The listing builds one solid part. Answer for the finished solid, in the listing's coordinates (mm). A direction names the side the tool comes from. Give positions to 0.01 mm unless a question says otherwise; leave off trailing zeros. Write each loop counter-clockwise with the first axis right and the second up, starting at its lowest first coordinate (ties: lowest second). Pieces come first, ordered by that corner, then holes. Notation, with made-up numbers: (71, -37.5) -> (96, -37.5) arc R12 ccw to (96, -30.5) -> close; hole circle Ø11 at (24.5, 50). An arc over 180 degrees is marked (long way). One line per question, with ' | ' between items.
from build123d import *

# Parameters (mm, degrees)
SKETCH1_W           = 43
SKETCH1_H           = 21
BOSS_EXTRUDE1_DEPTH = 1.2
SKETCH2_R           = 0.5
CUT_EXTRUDE1_DEPTH  = 48.868987873
SKETCH3_R           = 1.5
CUT_EXTRUDE2_DEPTH  = 48.868987873
SKETCH4_W           = 9.5
SKETCH4_H           = 4.82
BOSS_EXTRUDE2_DEPTH = 11.88
SKETCH5_R           = 1.12
BOSS_EXTRUDE3_DEPTH = 1.6
SKETCH6_W           = 7.46
SKETCH6_H           = 2.45
BOSS_EXTRUDE4_DEPTH = 0.6
SKETCH7_W           = 12.24
SKETCH7_H           = 12.24
BOSS_EXTRUDE5_DEPTH = 7.61
SKETCH8_W           = 10.2
SKETCH8_H           = 12.8
BOSS_EXTRUDE6_DEPTH = 5.8
SKETCH9_W           = 5.4
SKETCH9_H           = 2.7
BOSS_EXTRUDE7_DEPTH = 2.05
SKETCH10_R          = 4.12
BOSS_EXTRUDE8_DEPTH = 10.3
SKETCH11_R          = 4
BOSS_EXTRUDE9_DEPTH = 10.5


with BuildPart() as part:
    # Sketch1 → Boss-Extrude1 (new body)
    with BuildSketch(Plane(origin=(0, 0, 0), x_dir=(1, 0, 0), z_dir=(0, 1, 0))):
        with Locations((21.5, 10.5)):
            Rectangle(SKETCH1_W, SKETCH1_H)
    extrude(amount=BOSS_EXTRUDE1_DEPTH)

    # Sketch2 → Cut-Extrude1 (cut, through all)
    with BuildSketch(Plane(origin=(0, 1.2, 0), x_dir=(1, 0, 0), z_dir=(0, 1, 0))):
        with Locations(Location((1.4, 19.3, 0), (0, 0, 270))):
            Circle(SKETCH2_R)
        with Locations(Location((1.4, 1.5, 0), (0, 0, 270))):
            Circle(SKETCH2_R)
        with Locations(Location((41.6, 19.3, 0), (0, 0, 270))):
            Circle(SKETCH2_R)
        with Locations(Location((41.6, 1.5, 0), (0, 0, 270))):
            Circle(SKETCH2_R)
    extrude(amount=-CUT_EXTRUDE1_DEPTH, mode=Mode.SUBTRACT)

    # Sketch3 → Cut-Extrude2 (cut, through all)
    with BuildSketch(Plane(origin=(0, 1.2, 0), x_dir=(1, 0, 0), z_dir=(0, 1, 0))):
        with Locations(Location((5.9, 18.94, 0), (0, 0, 270))):
            Circle(SKETCH3_R)
        with Locations(Location((37.05, 2.23, 0), (0, 0, 270))):
            Circle(SKETCH3_R)
    extrude(amount=-CUT_EXTRUDE2_DEPTH, mode=Mode.SUBTRACT)

    # Sketch4 → Boss-Extrude2 (add)
    with BuildSketch(Plane(origin=(0, 1.2, 0), x_dir=(1, 0, 0), z_dir=(0, 1, 0))):
        with Locations((28.93, 18.49)):
            Rectangle(SKETCH4_W, SKETCH4_H)
    extrude(amount=BOSS_EXTRUDE2_DEPTH)

    # Sketch5 → Boss-Extrude3 (add)
    with BuildSketch(Plane(origin=(0, 13.08, 0), x_dir=(1, 0, 0), z_dir=(0, 1, 0))):
        with Locations(Location((25.3, 19.78, 0), (0, 0, 90))):
            Circle(SKETCH5_R)
    extrude(amount=BOSS_EXTRUDE3_DEPTH)

    # Sketch6 → Boss-Extrude4 (add)
    with BuildSketch(Plane.XZ):
        with Locations((29.47, -18.275)):
            Rectangle(SKETCH6_W, SKETCH6_H)
    extrude(amount=BOSS_EXTRUDE4_DEPTH)

    # Sketch7 → Boss-Extrude5 (add)
    with BuildSketch(Plane(origin=(0, 1.2, 0), x_dir=(1, 0, 0), z_dir=(0, 1, 0))):
        with Locations((27.32, 6.87)):
            Rectangle(SKETCH7_W, SKETCH7_H)
    extrude(amount=BOSS_EXTRUDE5_DEPTH)

    # Sketch8 → Boss-Extrude6 (add)
    with BuildSketch(Plane(origin=(0, 1.2, 0), x_dir=(1, 0, 0), z_dir=(0, 1, 0))):
        with Locations((15.3, 13.5)):
            Rectangle(SKETCH8_W, SKETCH8_H)
    extrude(amount=BOSS_EXTRUDE6_DEPTH)

    # Sketch9 → Boss-Extrude7 (add)
    with BuildSketch(Plane(origin=(0, 1.2, 0), x_dir=(1, 0, 0), z_dir=(0, 1, 0))):
        with Locations((13.6, 2)):
            Rectangle(SKETCH9_W, SKETCH9_H)
    extrude(amount=BOSS_EXTRUDE7_DEPTH)

    # Sketch10 → Boss-Extrude8 (add)
    with BuildSketch(Plane(origin=(0, 1.2, 0), x_dir=(1, 0, 0), z_dir=(0, 1, 0))):
        with Locations(Location((4.62, 11.5, 0), (0, 0, 90))):
            Circle(SKETCH10_R)
    extrude(amount=BOSS_EXTRUDE8_DEPTH)

    # Sketch11 → Boss-Extrude9 (add)
    with BuildSketch(Plane(origin=(0, 1.2, 0), x_dir=(1, 0, 0), z_dir=(0, 1, 0))):
        with Locations(Location((38.28, 11.6, 0), (0, 0, 90))):
            Circle(SKETCH11_R)
    extrude(amount=BOSS_EXTRUDE9_DEPTH)


solid = part.part
Item 1: Find section D-D (z = -4.25). Write down the section's boundary in (x, y), then the cut area to 3 significant figures.
Answers below:
outline: (0, 0) -> (43, 0) -> (43, 1.2) -> (33.44, 1.2) -> (33.44, 8.81) -> (21.2, 8.81) -> (21.2, 1.2) -> (0, 1.2) -> close | area: 145 mm²
Item 2: A tool of negligible diameter and unlimited length cuts with its end or side. For faces 5 (the face through (25.25, 13.87, -18.66)), 6 (the face through (33.44, 5, -7)), 7 (the face through (14, 3.25, -2)), 8 (the face through (14, 2, -0.65)), from which of +Z, -Z, +X, -X, +Y, -Y can it reach the whole face along a straight path? Write none if from no direction.
Answers below:
face 5: +Y | face 6: +Z, +Y | face 7: +Z, -X, +Y | face 8: +Z, +X, -X, +Y
Item 3: Determine the mould class of faces 1 (the face through (38, 11.7, -12)), 2 (the face through (42, 1, -19)), 3 (the face through (27, 5, -0.75)), 4 (the face through (29, 7, -16.08)) for opening direction Z: pulls with the +Z half, pulls with the -Z half, needs draft (parallel to the pull), parting line crosses it, or undercut.
Answers below:
face 1: needs draft | face 2: undercut | face 3: pulls with the +Z half | face 4: undercut
Item 4: Flat-ended cylindrical pins translate along their axes: pin 1 (8 mm diameter, centred on x = 15.5, z = -11.5, fed in from +Y); pin 2 (5 mm diameter, centred on y = 13, z = -15, fed in from +X); pin 3 (1.7 mm diameter, centred on y = 3, z = -14, fed in from +X); pin 4 (2.5 mm diameter, centred on x = 37.05, z = -2.23, fed in from +Y). Find the tip coordinate at first contact, or state that the pin passes through.
Answers below:
pin 1: y = 7 | pin 2: x = 42.07 | pin 3: x = 41.97 | pin 4: through
Item 5: Find section C-C (z = -18). Write down the section's boundary in (x, y).
Answers below:
outline: (0, 0) -> (4.73, 0) -> (4.73, 1.2) -> (0, 1.2) -> close; (7.07, 0) -> (25.74, 0) -> (25.74, -0.6) -> (33.2, -0.6) -> (33.2, 0) -> (43, 0) -> (43, 1.2) -> (33.68, 1.2) -> (33.68, 13.08) -> (24.18, 13.08) -> (24.18, 1.2) -> (20.4, 1.2) -> (20.4, 7) -> (10.2, 7) -> (10.2, 1.2) -> (7.07, 1.2) -> close
Item 6: Consider line 1 (X direction, y = 5.5, z = -8.25); line 2 (X direction, y = 0.5, z = -1.5); line 3 (X direction, y = 4, z = -14). Determine where each line is inside the solid, lowest interval first. Write a range as [from, to].
Answers below:
line 1: [2.09, 7.15], [10.2, 20.4], [21.2, 33.44], [36.09, 40.47] | line 2: [0, 0.9], [1.9, 35.74], [38.36, 41.1], [42.1, 43] | line 3: [1.35, 7.89], [10.2, 20.4], [35.08, 41.48]
Item 7: Find section B-B (x = 22.5). Write down the section's boundary in (y, z), then the cut area to 3 significant figures.
Answers below:
outline: (0, -21) -> (1.2, -21) -> (1.2, -12.99) -> (8.81, -12.99) -> (8.81, -0.75) -> (1.2, -0.75) -> (1.2, 0) -> (0, 0) -> close | area: 118 mm²
Item 8: Find section A-A (y = 2.75). Write down the section's boundary in (x, z), then the cut area to 3 significant figures.
Answers below:
outline: circle Ø8.24 at (4.62, -11.5); (10.2, -19.9) -> (20.4, -19.9) -> (20.4, -7.1) -> (10.2, -7.1) -> close; (10.9, -3.35) -> (16.3, -3.35) -> (16.3, -0.65) -> (10.9, -0.65) -> close; (21.2, -12.99) -> (33.44, -12.99) -> (33.44, -0.75) -> (21.2, -0.75) -> close; (24.18, -20.9) -> (33.68, -20.9) -> (33.68, -16.08) -> (24.18, -16.08) -> close; circle Ø8 at (38.28, -11.6) | area: 444 mm²
